from build123d import *

# Parameters (mm, degrees)
F0_W        = 40
F0_H        = 20
F0_R        = 2.0889371437
F1_DEPTH    = 4
F2_T1_DEPTH = 65.7168298797
F2_T3_DEPTH = 45.7168298797


# Not quite as in the source:
# - a fillet or chamfer that OpenCascade refuses, or shapes differently, is made with other operations: its cross-section is extruded or revolved along the edge and cut away or added


with BuildPart() as f1:
    # F0 (on Top) → F1 (new body)
    with BuildSketch(Plane.XY):
        with Locations((20, 10)):
            Rectangle(F0_W, F0_H)
        Polygon((11.590113647, 5.4027722217), (7.3983091854, 5.4027722217), (7.3983091854, 12.1895739882), (8.8376637294, 12.1895739882), (8.8376637294, 6.5910938267), (11.590113647, 6.5910938267), align=None, mode=Mode.SUBTRACT)
        with BuildLine():
            Line((17.4203165215, 5.4027722217), (16.3344876549, 5.4027722217))
            Line((16.3344876549, 5.4027722217), (16.1443561981, 6.0667469185))
            Line((16.1443561981, 6.0667469185), (16.0700860978, 6.0667469185))
            add(Edge.make_bspline(
                [(16.0700860978, 6.0667469185), (15.8428195908, 5.704308829), (15.4246789261, 5.5067503622)],
                knots=[0, 0, 0, 1, 1, 1], degree=2))
            add(Edge.make_bspline(
                [(15.4246789261, 5.5067503622), (15.0065382613, 5.3091918953), (14.4732789411, 5.3091918953)],
                knots=[0, 0, 0, 1, 1, 1], degree=2))
            add(Edge.make_bspline(
                [(14.4732789411, 5.3091918953), (13.5582713053, 5.3091918953), (13.0940831783, 5.7993745574)],
                knots=[0, 0, 0, 1, 1, 1], degree=2))
            add(Edge.make_bspline(
                [(13.0940831783, 5.7993745574), (12.6298950514, 6.2895572194), (12.6298950514, 7.2090210613)],
                knots=[0, 0, 0, 1, 1, 1], degree=2))
            Line((12.6298950514, 7.2090210613), (12.6298950514, 10.5927668315))
            Line((12.6298950514, 10.5927668315), (14.0454831633, 10.5927668315))
            Line((14.0454831633, 10.5927668315), (14.0454831633, 7.5610613368))
            add(Edge.make_bspline(
                [(14.0454831633, 7.5610613368), (14.0454831633, 6.9995793784), (14.2452697331, 6.7188383992)],
                knots=[0, 0, 0, 1, 1, 1], degree=2))
            add(Edge.make_bspline(
                [(14.2452697331, 6.7188383992), (14.445056303, 6.4380974201), (14.8817644928, 6.4380974201)],
                knots=[0, 0, 0, 1, 1, 1], degree=2))
            add(Edge.make_bspline(
                [(14.8817644928, 6.4380974201), (15.4759252953, 6.4380974201), (15.7403268524, 6.8346997557)],
                knots=[0, 0, 0, 1, 1, 1], degree=2))
            add(Edge.make_bspline(
                [(15.7403268524, 6.8346997557), (16.0047284095, 7.2313020914), (16.0047284095, 8.1507659333)],
                knots=[0, 0, 0, 1, 1, 1], degree=2))
            Line((16.0047284095, 8.1507659333), (16.0047284095, 10.5927668315))
            Line((16.0047284095, 10.5927668315), (17.4203165215, 10.5927668315))
            Line((17.4203165215, 10.5927668315), (17.4203165215, 5.4027722217))
        make_face(mode=Mode.SUBTRACT)
        with BuildLine():
            Line((23.6961399978, 8.7865179919), (23.6961399978, 5.4027722217))
            Line((23.6961399978, 5.4027722217), (22.2805518859, 5.4027722217))
            Line((22.2805518859, 5.4027722217), (22.2805518859, 8.4344777164))
            add(Edge.make_bspline(
                [(22.2805518859, 8.4344777164), (22.2805518859, 8.9959596748), (22.080765316, 9.276700654)],
                knots=[0, 0, 0, 1, 1, 1], degree=2))
            add(Edge.make_bspline(
                [(22.080765316, 9.276700654), (21.8809787462, 9.5574416332), (21.4442705564, 9.5574416332)],
                knots=[0, 0, 0, 1, 1, 1], degree=2))
            add(Edge.make_bspline(
                [(21.4442705564, 9.5574416332), (20.8501097539, 9.5574416332), (20.5857081968, 9.1608392975)],
                knots=[0, 0, 0, 1, 1, 1], degree=2))
            add(Edge.make_bspline(
                [(20.5857081968, 9.1608392975), (20.3213066396, 8.7642369618), (20.3213066396, 7.84477312)],
                knots=[0, 0, 0, 1, 1, 1], degree=2))
            Line((20.3213066396, 7.84477312), (20.3213066396, 5.4027722217))
            Line((20.3213066396, 5.4027722217), (18.9057185277, 5.4027722217))
            Line((18.9057185277, 5.4027722217), (18.9057185277, 10.5927668315))
            Line((18.9057185277, 10.5927668315), (19.9870911882, 10.5927668315))
            Line((19.9870911882, 10.5927668315), (20.177222645, 9.9287921347))
            Line((20.177222645, 9.9287921347), (20.2559489514, 9.9287921347))
            add(Edge.make_bspline(
                [(20.2559489514, 9.9287921347), (20.4936132724, 10.3045988423), (20.9087831331, 10.4969584021)],
                knots=[0, 0, 0, 1, 1, 1], degree=2))
            add(Edge.make_bspline(
                [(20.9087831331, 10.4969584021), (21.3239529939, 10.6893179619), (21.8527561081, 10.6893179619)],
                knots=[0, 0, 0, 1, 1, 1], degree=2))
            add(Edge.make_bspline(
                [(21.8527561081, 10.6893179619), (22.7588513319, 10.6893179619), (23.2274956648, 10.1998780009)],
                knots=[0, 0, 0, 1, 1, 1], degree=2))
            add(Edge.make_bspline(
                [(23.2274956648, 10.1998780009), (23.6961399978, 9.7104380398), (23.6961399978, 8.7865179919)],
                knots=[0, 0, 0, 1, 1, 1], degree=2))
        make_face(mode=Mode.SUBTRACT)
        with BuildLine():
            Line((29.4372187519, 5.4027722217), (28.4494264178, 5.4027722217))
            Line((28.4494264178, 5.4027722217), (28.1746270466, 6.1083381747))
            Line((28.1746270466, 6.1083381747), (28.1374919965, 6.1083381747))
            add(Edge.make_bspline(
                [(28.1374919965, 6.1083381747), (27.780995515, 5.6582613668), (27.4022180034, 5.4837266311)],
                knots=[0, 0, 0, 1, 1, 1], degree=2))
            add(Edge.make_bspline(
                [(27.4022180034, 5.4837266311), (27.0234404918, 5.3091918953), (26.4159110712, 5.3091918953)],
                knots=[0, 0, 0, 1, 1, 1], degree=2))
            add(Edge.make_bspline(
                [(26.4159110712, 5.3091918953), (25.6687538621, 5.3091918953), (25.2394726823, 5.7369876731)],
                knots=[0, 0, 0, 1, 1, 1], degree=2))
            add(Edge.make_bspline(
                [(25.2394726823, 5.7369876731), (24.8101915025, 6.1647834509), (24.8101915025, 6.9535319162)],
                knots=[0, 0, 0, 1, 1, 1], degree=2))
            add(Edge.make_bspline(
                [(24.8101915025, 6.9535319162), (24.8101915025, 7.7794154317), (25.3880128829, 8.1715615613)],
                knots=[0, 0, 0, 1, 1, 1], degree=2))
            add(Edge.make_bspline(
                [(25.3880128829, 8.1715615613), (25.9658342633, 8.563707691), (27.1303894362, 8.6052989472)],
                knots=[0, 0, 0, 1, 1, 1], degree=2))
            Line((27.1303894362, 8.6052989472), (28.032028454, 8.6335215853))
            Line((28.032028454, 8.6335215853), (28.032028454, 8.8607880922))
            add(Edge.make_bspline(
                [(28.032028454, 8.8607880922), (28.032028454, 9.6495365575), (27.2239697626, 9.6495365575)],
                knots=[0, 0, 0, 1, 1, 1], degree=2))
            add(Edge.make_bspline(
                [(27.2239697626, 9.6495365575), (26.601586322, 9.6495365575), (25.7608487865, 9.27372985)],
                knots=[0, 0, 0, 1, 1, 1], degree=2))
            Line((25.7608487865, 9.27372985), (25.2929471545, 10.230328742))
            add(Edge.make_bspline(
                [(25.2929471545, 10.230328742), (26.1886445643, 10.699715776), (27.2789296369, 10.699715776)],
                knots=[0, 0, 0, 1, 1, 1], degree=2))
            add(Edge.make_bspline(
                [(27.2789296369, 10.699715776), (28.3231672472, 10.699715776), (28.8801929996, 10.244440061)],
                knots=[0, 0, 0, 1, 1, 1], degree=2))
            add(Edge.make_bspline(
                [(28.8801929996, 10.244440061), (29.4372187519, 9.7891643461), (29.4372187519, 8.8607880922)],
                knots=[0, 0, 0, 1, 1, 1], degree=2))
            Line((29.4372187519, 8.8607880922), (29.4372187519, 5.4027722217))
        make_face(mode=Mode.SUBTRACT)
        with Locations((18.9712941647, 16.7298167944)):
            Circle(F0_R, mode=Mode.SUBTRACT)
    extrude(amount=F1_DEPTH)

    # F2: chamfer of 5 on 4 edges, made by hand

    # F2_s2 → F2_t1 (cut)
    with BuildSketch(Plane.YZ.offset(-12.8584149398)):
        Polygon((20, -1), (15, 4), (20, 4), align=None)
        Polygon((0, -1), (5, 4), (0, 4), align=None)
    extrude(amount=F2_T1_DEPTH, mode=Mode.SUBTRACT)

    # F2_s4 → F2_t3 (cut)
    with BuildSketch(Plane.XZ.offset(-32.8584149398)):
        Polygon((0, -1), (5, 4), (0, 4), align=None)
        Polygon((40, -1), (35, 4), (40, 4), align=None)
    extrude(amount=F2_T3_DEPTH, mode=Mode.SUBTRACT)


solid = f1.part
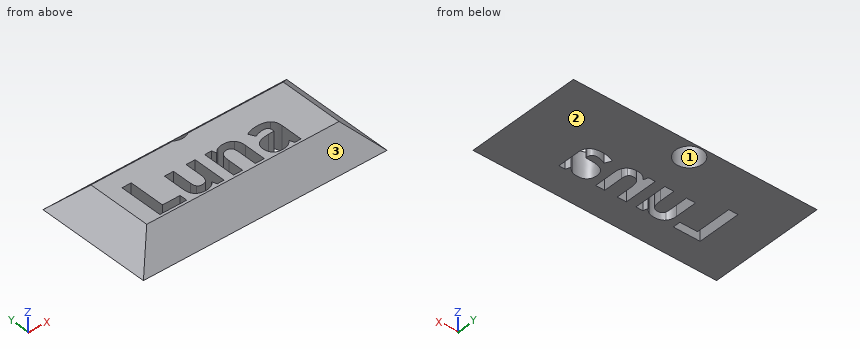
Build history of the part. All positions in model axes, mm. Face numbers are marked on the shaded views. Round coordinates to 2 decimals unless told otherwise and drop trailing zeros. Loops run counter-clockwise (first coordinate to the right, second up) from the corner with the lowest first, then second, coordinate; pieces in that order, holes last. Notation, with made-up numbers: (22.5, 39.5) -> (43.5, 39.5) arc R17 ccw to (43.5, 56.5) -> close; hole circle Ø2 at (54, 3.5). An arc over 180 degrees is marked (long way). One line per item, written item: value. Start each with the question number.
Q1. Cut at C-C on x = 30. List the corners of the cut face in (y, z).
Q2. Drop flat-ended pins along their axis: pin 1 Ø0.9 at (y, z) = (6.5, 2.5) entering from +X; pin 2 Ø2 at (x, z) = (10.5, 2.5) entering from -Y; pin 3 Ø0.5 at (x, z) = (29, 1.5) entering from +Y. Give the stop position or say it passes through.
Q3. Cut at B-B on y = 13.75. List the corners of the cut face in (x, z).
Q4. Cut at D-D on z = 1.7. Count the separate pieces of the cut face and the enclosed holes in it, plus the area to 3 significant figures.
Q5. Cut at A-A on x = 10. List the corners of the cut face in (y, z), plus the area to 3 significant figures.
Q6. Probe line 1 along Y through (x, z) = (26.5, 0.7); line 2 along Y through (x, z) = (13, 3.65); line 3 along X through (y, z) = (15.5, 0.75). List the from-to ranges inside material, lowest first.
Q7. Two-plate mould, pull along Y, no slides. Class the marked faces 1, 2 and 3: released by +Y, released by -Y, zero draft, split by the parting line, or undercut.
Computed:
1. outline: (1, 0) -> (19, 0) -> (15, 4) -> (5, 4) -> close
2. pin 1: x = 36.95
2. pin 2: y = 2.5
2. pin 3: y = 17.75
3. outline: (1, 0) -> (39, 0) -> (35, 4) -> (5, 4) -> close
4. separate pieces: 1
4. enclosed holes: 4
4. area: 431 mm²
5. outline: (1, 0) -> (5.4, 0) -> (5.4, 4) -> (5, 4) -> close; (6.59, 0) -> (19, 0) -> (15, 4) -> (6.59, 4) -> close
5. area: 51.2 mm²
6. line 1: 1.7 to 5.31, 8.55 to 9.54, 10.64 to 18.3
6. line 2: 4.65 to 5.91, 10.59 to 15.35
6. line 3: 1.75 to 17.28, 20.66 to 38.25
7. face 1: undercut
7. face 2: zero draft
7. face 3: released by -Y
